Check sheet for the modelled part. Datum: model origin and axes. Units: mm. A direction names the side the tool comes from. Give positions to 0.01 mm unless a question says otherwise; leave off trailing zeros. Order: outer loops, then holes, each group sorted by start corner. A loop starts at its lowest first (then second) coordinate and runs counter-clockwise, first axis right, second up. Notation, with made-up numbers: (77, 83) - (120, 83) arc R21 cw to (120, 97) - close; hole circle Ø11 at (2.25, 37). An arc over 180 degrees is marked (long way). Answer in a Markdown table with one row per item.
from build123d import *

# Parameters (mm, degrees)
F0_W     = 31.75
F0_H     = 7.9375
F1_DEPTH = 11.1125
F2_W     = 9.525
F2_H     = 7.9375
F3_DEPTH = 9.525
F4_W     = 4.7625
F4_H     = 9.525
F5_DEPTH = 22.226


# Not quite as in the source:
# - a length typed as a fraction of an inch, garbled in the dataset ("3 / 203.2 mm" for 3/8 in), is restored


with BuildPart() as f1:
    # F0 (on Top) → F1 (new body)
    with BuildSketch(Plane.XY):
        with Locations((-0.0819904208, 12.7078423367)):
            Rectangle(F0_W, F0_H)
    extrude(amount=F1_DEPTH)

    # F2 (on face) → F3 (cut)
    with BuildSketch(Plane.XY.offset(11.1125)):
        with Locations((11.0305095792, 12.7078423367)):
            Rectangle(F2_W, F2_H)
    extrude(amount=-F3_DEPTH, mode=Mode.SUBTRACT)

    # F4 (on face) → F5 (cut, through all)
    with BuildSketch(Plane.YZ.offset(6.2680095792)):
        with Locations((12.7078423367, 6.35)):
            Rectangle(F4_W, F4_H)
    extrude(amount=-F5_DEPTH, mode=Mode.SUBTRACT)


solid = f1.part
(1) Cross-section at C-C, the plane y = 15.5. Record the cut outline in (x, z).
Geometry says:
| item | result |
|---|---|
| outline | (-15.96, 0) - (15.79, 0) - (15.79, 1.59) - (6.27, 1.59) - (6.27, 11.11) - (-15.96, 11.11) - close |
(2) Cross-section at A-A, the plane z = 10. Record the cut outline in (x, y), then the cut area to 3 significant figures.
Geometry says:
| item | result |
|---|---|
| outline | (-15.96, 8.74) - (6.27, 8.74) - (6.27, 10.33) - (-15.96, 10.33) - close; (-15.96, 15.09) - (6.27, 15.09) - (6.27, 16.68) - (-15.96, 16.68) - close |
| area | 70.6 mm² |
(3) Cross-section at B-B, the plane x = -10. Record the cut outline in (y, z).
Geometry says:
| item | result |
|---|---|
| outline | (8.74, 0) - (16.68, 0) - (16.68, 11.11) - (15.09, 11.11) - (15.09, 1.59) - (10.33, 1.59) - (10.33, 11.11) - (8.74, 11.11) - close |
(4) Gauge pin test, flat ends, axial feed: P1, Ø1.5, axis at x = -8, y = 12.5, coming from the +Z side; P2, Ø1.3, axis at y = 10, z = 8.5, coming from the +X side. Record the tip position at first contact, or that the pin passes through.
Geometry says:
| item | result |
|---|---|
| P1 | z = 1.59 |
| P2 | x = 6.27 |
(5) Mould release check, pull along Y, two halves, no side actions. Record for faces 1 (the flat face through (-4, 16.677, 5)), 2 (the flat face through (-4, 8.739, 5)), 3 (the flat face through (-5, 16, 11.112)), 4 (the flat face through (-5, 15.089, 6)): pulls with the +Y half, pulls with the -Y half, needs draft (parallel to the pull), parting line crosses it, or undercut.
Geometry says:
| item | result |
|---|---|
| face 1 | pulls with the +Y half |
| face 2 | pulls with the -Y half |
| face 3 | needs draft |
| face 4 | undercut |
(6) Thickness scan on L1, parallel to Y at x = -4.5, z = 7.75; L2, parallel to Z at x = 14.5, y = 12.75; L3, parallel to X at y = 16, z = 10. Record the ranges inside material, lowest first.
Geometry says:
| item | result |
|---|---|
| L1 | 8.74 to 10.33, 15.09 to 16.68 |
| L2 | 0 to 1.59 |
| L3 | -15.96 to 6.27 |
(7) Cross-section at D-D, the plane y = 13.25. Record the cut outline in (x, z), then the cut area to 3 significant figures.
Geometry says:
| item | result |
|---|---|
| outline | (-15.96, 0) - (15.79, 0) - (15.79, 1.59) - (-15.96, 1.59) - close |
| area | 50.4 mm² |
(8) Access from +Z, -Z, +X, -X, +Y, -Y to the whole of each face (thin tool, end or side, straight path). Record for faces 5 (the flat face through (0, 13, 0)), 6 (the flat face through (6.268, 10, 6)), 7 (the flat face through (-5, 10.327, 6)).
Geometry says:
| item | result |
|---|---|
| face 5 | -Z, +X, -X, +Y, -Y |
| face 6 | +Z, +X, +Y, -Y |
| face 7 | +Z, +X, -X |
